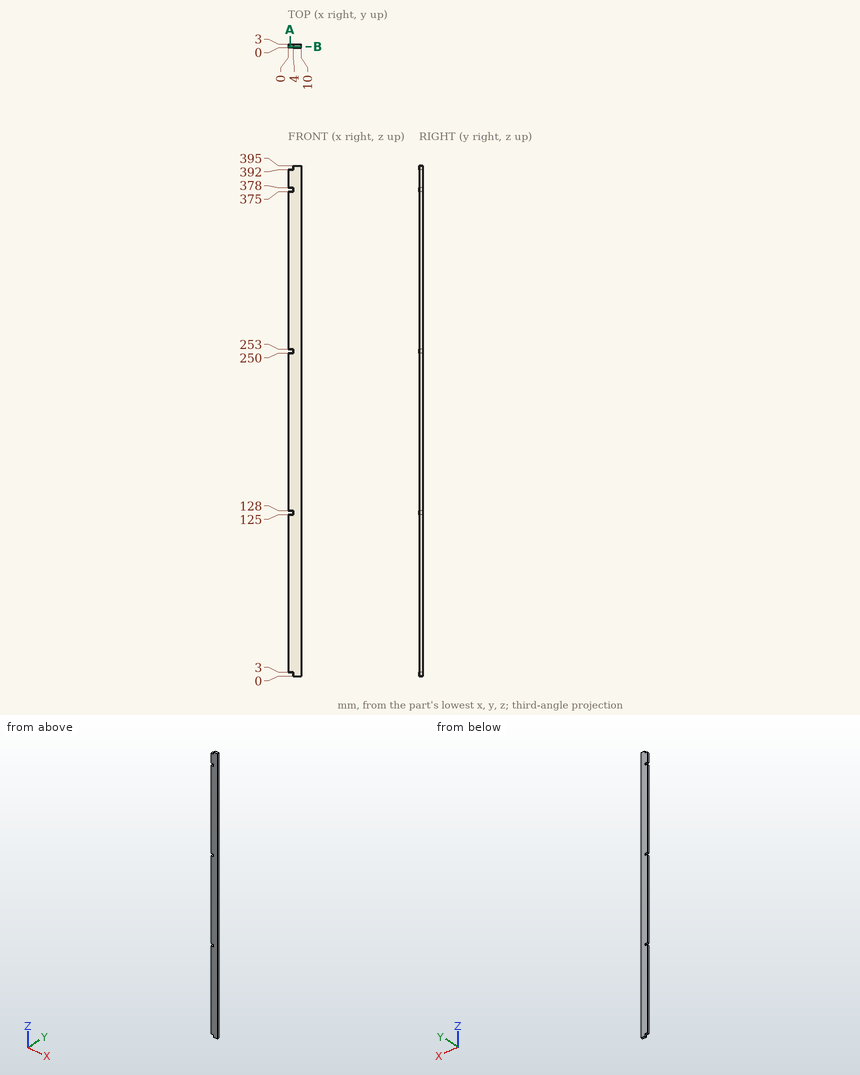
Geometry check sheet. Reference: drawing and pictorial views, mm from the part's lowest x, y, z. Coordinates: 2 decimals unless noted, no trailing zeros. Order: outer loops, then holes, each group sorted by start corner. A loop starts at its lowest first (then second) coordinate and runs counter-clockwise, first axis right, second up.
Item 1: Depth check by flat-ended pin: pin 1 (0.9 mm diameter, centred on x = 1.5, y = 1, fed in from -Z); pin 2 (0.9 mm diameter, centred on x = 2, y = 2, fed in from +Z); pin 3 (1.5 mm diameter, centred on y = 2, z = 394, fed in from -X). Enter the tip coordinate at first touch or a pass-through.
Filled in:
pin 1: stops at z = 3
pin 2: stops at z = 392
pin 3: stops at x = 4
Item 2: Material ranges on L1, parallel to Z at x = 0.5, y = 2.05, recorded low to high.
Filled in:
L1: z = 3 to 125, 128 to 250, 253 to 375, 378 to 392
Item 3: Section check A-A, the plane x = 1.5. Enter the section's corners in (y, z), then the cut area to 3 significant figures.
Filled in:
outline: (0, 3) - (3, 3) - (3, 125) - (0, 125) - close; (0, 128) - (3, 128) - (3, 250) - (0, 250) - close; (0, 253) - (3, 253) - (3, 375) - (0, 375) - close; (0, 378) - (3, 378) - (3, 392) - (0, 392) - close
area: 1,140 mm2
Item 4: Section check B-B, the plane y = 1. Enter the section's corners in (x, z).
Filled in:
outline: (0, 3) - (4, 3) - (4, 0) - (10, 0) - (10, 395) - (4, 395) - (4, 392) - (0, 392) - (0, 378) - (4, 378) - (4, 375) - (0, 375) - (0, 253) - (4, 253) - (4, 250) - (0, 250) - (0, 128) - (4, 128) - (4, 125) - (0, 125) - close
